```python
from build123d import *

# Parameters (mm, degrees)
BOSS_EXTRUDE1_DEPTH     = 3
CUT_EXTRUDE1_DEPTH      = 38.656340768
CUT_EXTRUDE1_DEPTH_BACK = 38.656340768
SKETCH2_W               = 39.2
SKETCH2_H               = 19.4
CUT_EXTRUDE2_DEPTH      = 38.656340768
CUT_EXTRUDE2_DEPTH_BACK = 38.656340768
SKETCH3_R               = 1.3
CUT_EXTRUDE3_DEPTH      = 2
SKETCH5_W               = 50
SKETCH5_H               = 15
BOSS_EXTRUDE2_DEPTH     = 3


with BuildPart() as part:
    # Sketch1 → Boss-Extrude1 (new body)
    with BuildSketch(Plane.XY):
        with BuildLine():
            Line((-23, -28), (23, -28))
            ThreePointArc((23, -28), (24.414213562, -27.414213562), (25, -26))
            Line((25, -26), (25, -2))
            ThreePointArc((25, -2), (24.414213562, -0.585786438), (23, 0))
            Line((23, 0), (-23, 0))
            ThreePointArc((-23, 0), (-24.414213562, -0.585786438), (-25, -2))
            Line((-25, -2), (-25, -26))
            ThreePointArc((-25, -26), (-24.414213562, -27.414213562), (-23, -28))
        make_face()
    extrude(amount=BOSS_EXTRUDE1_DEPTH)

    # Sketch2 → Cut-Extrude1 (cut, two sides: drawn at the far end of the back side and taken through both)
    with BuildSketch(Plane.XY.offset(-CUT_EXTRUDE1_DEPTH_BACK)):
        with Locations((0, -10.9)):
            Rectangle(SKETCH2_W, SKETCH2_H)
    extrude(amount=CUT_EXTRUDE1_DEPTH + CUT_EXTRUDE1_DEPTH_BACK, mode=Mode.SUBTRACT)

    # Sketch3 → Cut-Extrude2 (cut, two sides: drawn at the far end of the back side and taken through both)
    with BuildSketch(Plane.XY.offset(-CUT_EXTRUDE2_DEPTH_BACK)):
        with Locations((23, -5.9)):
            Circle(SKETCH3_R)
        with Locations((23, -15.9)):
            Circle(SKETCH3_R)
        with Locations((-23, -5.9)):
            Circle(SKETCH3_R)
        with Locations((-23, -15.9)):
            Circle(SKETCH3_R)
    extrude(amount=CUT_EXTRUDE2_DEPTH + CUT_EXTRUDE2_DEPTH_BACK, mode=Mode.SUBTRACT)

    # Sketch4 → Cut-Extrude3 (cut)
    with BuildSketch(Plane.XY):
        Polygon((25.1, -4.687564435), (23, -3.475128869), (20.9, -4.687564435), (20.9, -7.112435565), (23, -8.324871131), (25.1, -7.112435565), align=None)
        Polygon((25.1, -14.687564435), (23, -13.475128869), (20.9, -14.687564435), (20.9, -17.112435565), (23, -18.324871131), (25.1, -17.112435565), align=None)
        Polygon((-20.9, -4.687564435), (-23, -3.475128869), (-25.1, -4.687564435), (-25.1, -7.112435565), (-23, -8.324871131), (-20.9, -7.112435565), align=None)
        Polygon((-20.9, -14.687564435), (-23, -13.475128869), (-25.1, -14.687564435), (-25.1, -17.112435565), (-23, -18.324871131), (-20.9, -17.112435565), align=None)
    extrude(amount=CUT_EXTRUDE3_DEPTH, mode=Mode.SUBTRACT)

    # Sketch5 → Boss-Extrude2 (add)
    with BuildSketch(Plane(origin=(0, 0, 0), x_dir=(1, 0, 0), z_dir=(0, 1, 0))):
        with Locations((0, 4.5)):
            Rectangle(SKETCH5_W, SKETCH5_H)
    extrude(amount=BOSS_EXTRUDE2_DEPTH)


solid = part.part
```
Verification items for the finished model (mm, model axes). A direction names the side the tool comes from. Coordinates: 2 decimals unless noted, no trailing zeros. Write each loop counter-clockwise with the first axis right and the second up, starting at its lowest first coordinate (ties: lowest second). Pieces come first, ordered by that corner, then holes. Notation, with made-up numbers: (70, -7) - (81, -7) arc R27 ccw to (81, 11) - close; hole circle Ø7 at (23.5, 29.25). An arc over 180 degrees is marked (long way). One line per question, with ' | ' between items. Start each with the question number.
1. Material ranges on line 1 along X through (y, z) = (-15.9, 2.4); line 2 along Y through (x, z) = (22.5, 1.5); line 3 along Y through (x, z) = (-21, -4), recorded low to high.
2. Section check A-A (y = -15.9). Enter the section's corners in (x, z), plus the area to 3 significant figures.
3. Access from +Z, -Z, +X, -X, +Y, -Y to the whole of each face (thin tool, end or side, straight path). Record for faces 4 (the flat face through (0, -1.2, 1)), 5 (the flat face through (24.01, -14.06, 0.99)), 6 (the flat face through (20.9, -16, 1)).
4. Draft check along X on faces 1 (the flat face through (25, 1, -4)), 2 (the flat face through (21.965, -14.073, 0.986)), 3 (the flat face through (0, 3, -5)). Enter one of: released by +X, released by -X, zero draft, split by the parting line, or undercut.
5. Section check B-B (x = -7). Enter the section's corners in (y, z), plus the area to 3 significant figures.
6. Gauge pin test, flat ends, axial feed: P1, Ø1, axis at y = -16, z = 1, coming from the -X side; P2, Ø8, axis at x = 16, y = -8.5, coming from the -Z side; P3, Ø1.2, axis at x = 23, y = -5, coming from the -Z side. Record the tip position at first contact, or that the pin passes through.
7. Section check D-D (z = -1.25). Enter the section's corners in (x, y), plus the area to 3 significant figures.
8. Section check C-C (y = -19.5). Enter the section's corners in (x, z).
Computed values:
1) line 1: -25 to -24.3, -21.7 to -19.6, 19.6 to 21.7, 24.3 to 25 | line 2: -28 to -18.04, -13.76 to -8.04, -3.76 to 3 | line 3: 0 to 3
2) outline: (-25, 2) - (-24.3, 2) - (-24.3, 3) - (-25, 3) - close; (-21.7, 2) - (-20.9, 2) - (-20.9, 0) - (-19.6, 0) - (-19.6, 3) - (-21.7, 3) - close; (19.6, 0) - (20.9, 0) - (20.9, 2) - (21.7, 2) - (21.7, 3) - (19.6, 3) - close; (24.3, 2) - (25, 2) - (25, 3) - (24.3, 3) - close | area: 10.8 mm²
3) face 4: +Z, -Z | face 5: -Z | face 6: -Z, +X
4) face 1: released by +X | face 2: undercut | face 3: zero draft
5) outline: (-28, 0) - (-20.6, 0) - (-20.6, 3) - (-28, 3) - close; (-1.2, 0) - (0, 0) - (0, -12) - (3, -12) - (3, 3) - (-1.2, 3) - close | area: 70.8 mm²
6) P1: x = -20.9 | P2: z = 0 | P3: z = 2
7) outline: (-25, 0) - (25, 0) - (25, 3) - (-25, 3) - close | area: 150 mm²
8) outline: (-25, 0) - (-19.6, 0) - (-19.6, 3) - (-25, 3) - close; (19.6, 0) - (25, 0) - (25, 3) - (19.6, 3) - close
